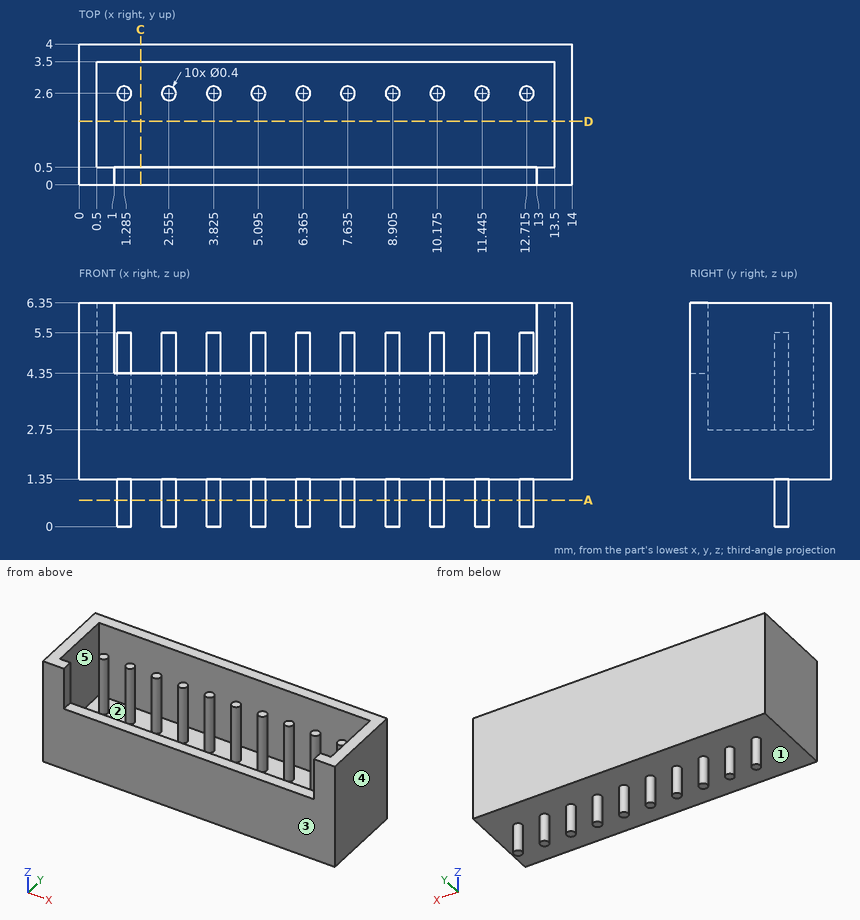
Study the drawing (mm; zero at the part's minimum x, y, z) and answer. A direction names the side the tool comes from. Coordinates: 2 decimals unless noted, no trailing zeros. Loops run counter-clockwise (first coordinate to the right, second up) from the corner with the lowest first, then second, coordinate; pieces in that order, holes last. Notation, with made-up numbers: (50, 47) -> (96, 47) arc R11 cw to (96, 57) -> close; hole circle Ø9 at (40.5, -16.75). An arc over 180 degrees is marked (long way). Write item = value, one per line. Start each with the question number.
1) The mould has two halves that part along Y. Classify the marked faces 1, 2 and 3: pulls with the +Y half, pulls with the -Y half, needs draft (parallel to the pull), parting line crosses it, or undercut.
2) The part is cut by section A-A, the plane z = 0.75. State how many separate pieces and enclosed holes the cut face has, plus the area to 3 significant figures.
3) The part is cut by section C-C, the plane x = 1.75. Determine the outline of the cut face in (y, z).
4) Find the intervals of material crossed by L1, parallel to X at y = 1.95, z = 4; L2, parallel to Y at x = 3.75, z = 3.5; L3, parallel to X at y = 0.35, z = 4.75, in increasing order. Write a range as from..to.
5) The part is cut by section D-D, the plane y = 1.8. Determine the outline of the cut face in (x, z).
6) Given P1, Ø1, axis at x = 2, y = 1.5, coming from the -Z side; P2, Ø0.9, axis at x = 8.5, y = 2, coming from the +Z side; P3, Ø0.6, axis at x = 8, y = 0.5, coming from the +Z side, each flat-ended and moving along its own axis, determine where each tip first touches the part or whether it passes through.
7) For the marked faces 4 and 5, determine the directions among +Z, -Z, +X, -X, +Y, -Y from which every point of the face is accessible in a straight line to the end or side of a thin tool.
Result:
q1.face_1 = needs draft
q1.face_2 = undercut
q1.face_3 = pulls with the -Y half
q2.separate_pieces = 10
q2.enclosed_holes = 0
q2.area = 1.26 mm²
q3.outline = (0, 1.35) -> (4, 1.35) -> (4, 6.35) -> (3.5, 6.35) -> (3.5, 2.75) -> (0.5, 2.75) -> (0.5, 4.35) -> (0, 4.35) -> close
q4.L1 = 0..0.5, 13.5..14
q4.L2 = 0..0.5, 2.41..2.79, 3.5..4
q4.L3 = 0..1, 13..14
q5.outline = (0, 1.35) -> (14, 1.35) -> (14, 6.35) -> (13.5, 6.35) -> (13.5, 2.75) -> (0.5, 2.75) -> (0.5, 6.35) -> (0, 6.35) -> close
q6.P1 = 1.35
q6.P2 = 2.75
q6.P3 = 4.35
q7.face_4 = +Z, -Z, +X, +Y, -Y
q7.face_5 = +Z
